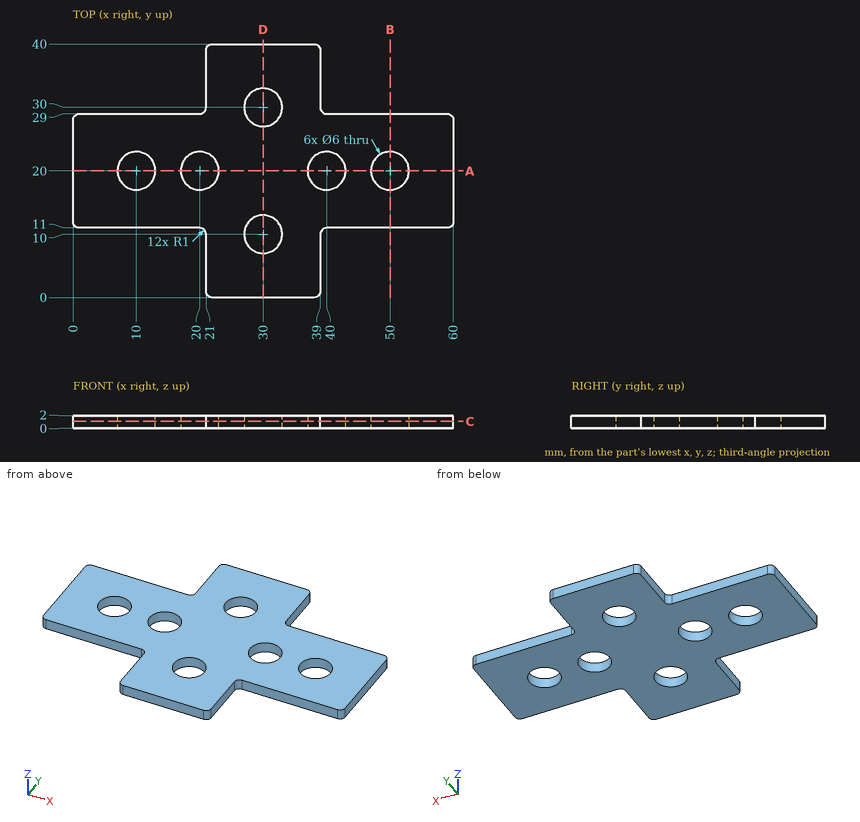
Design review of the part shown in the three views and the two pictorial views. Dimensions are in mm from the part's minimum x, y and z. Round coordinates to 2 decimals unless told otherwise and drop trailing zeros. Write each loop counter-clockwise with the first axis right and the second up, starting at its lowest first coordinate (ties: lowest second). Pieces come first, ordered by that corner, then holes.
Item 1: We need section C-C on z = 1.1. State how many separate pieces and enclosed holes the cut face has, and give its area (3 significant figures).
Item 2: We need section D-D on x = 30. Write out the cut boundary in (y, z).
Item 3: We need section A-A on y = 20. Write out the cut boundary in (x, z).
Item 4: We need section B-B on x = 50. Write out the cut boundary in (y, z), and give its area (3 significant figures).
Item 5: Clearance check with flat-ended pins moving along their axes: pin 1 Ø0.6 at (y, z) = (3.5, 0.5) entering from +X; pin 2 Ø0.6 at (x, z) = (51, 1.5) entering from -Y; pin 3 Ø1 at (x, y) = (39.5, 22.5) entering from -Z. State where each tip first meets the part, or that it passes through.
Item 6: For probe 1 along Y at (x, z) = (30, 1.2); probe 2 along Y at (x, z) = (50, 1.3); probe 3 along Y at (x, z) = (37.5, 1.7), list the stretches that pass through material, from the lowest coordinate up.
Returned:
1. separate pieces: 1
1. enclosed holes: 6
1. area: 1,310 mm2
2. outline: (0, 0) - (7, 0) - (7, 2) - (0, 2) - close; (13, 0) - (27, 0) - (27, 2) - (13, 2) - close; (33, 0) - (40, 0) - (40, 2) - (33, 2) - close
3. outline: (0, 0) - (7, 0) - (7, 2) - (0, 2) - close; (13, 0) - (17, 0) - (17, 2) - (13, 2) - close; (23, 0) - (37, 0) - (37, 2) - (23, 2) - close; (43, 0) - (47, 0) - (47, 2) - (43, 2) - close; (53, 0) - (60, 0) - (60, 2) - (53, 2) - close
4. outline: (11, 0) - (17, 0) - (17, 2) - (11, 2) - close; (23, 0) - (29, 0) - (29, 2) - (23, 2) - close
4. area: 24.0 mm2
5. pin 1: stops at x = 39
5. pin 2: stops at y = 11
5. pin 3: stops at z = 0
6. probe 1: y = 0 to 7, 13 to 27, 33 to 40
6. probe 2: y = 11 to 17, 23 to 29
6. probe 3: y = 0 to 18.34, 21.66 to 40
